from build123d import *

# Parameters (mm, degrees)
SKETCH1_W                 = 97.7
SKETCH1_H                 = 140
BOSS_EXTRUDE1_DEPTH       = 6.35
FILLET1_R                 = 10
CUT_EXTRUDE1_DEPTH        = 6.35
SKETCH5_R                 = 2.4
CUT_EXTRUDE2_DEPTH        = 6.35
F_5_0MM_DOWEL_HOLE1_D     = 5
F_5_0MM_DOWEL_HOLE1_DEPTH = 10
F_5_0MM_DOWEL_HOLE1_TIP   = 1.502151548


with BuildPart() as part:
    # Sketch1 → Boss-Extrude1 (new body)
    with BuildSketch(Plane(origin=(0, 0, 0), x_dir=(1, 0, 0), z_dir=(0, 1, 0))):
        with Locations((3.993769968, 7.891373802)):
            Rectangle(SKETCH1_W, SKETCH1_H)
    extrude(amount=BOSS_EXTRUDE1_DEPTH)

    # Fillet1
    fillet1_edges = [part.edges().sort_by_distance(p)[0] for p in [
        (-44.856230032, 3.175, -77.891373802),
        (-44.856230032, 3.175, 62.108626198),
    ]]
    fillet(fillet1_edges, radius=FILLET1_R)

    # Sketch3 → Cut-Extrude1 (cut)
    with BuildSketch(Plane(origin=(0, 6.35, 0), x_dir=(1, 0, 0), z_dir=(0, 1, 0))):
        Polygon((-29.556230032, 63.491373802), (-29.556230032, -40), (34.243769968, -40), (34.343769968, 63.391373802), align=None)
    extrude(amount=-CUT_EXTRUDE1_DEPTH, mode=Mode.SUBTRACT)

    # Sketch5 → Cut-Extrude2 (cut)
    with BuildSketch(Plane(origin=(0, 6.35, 0), x_dir=(1, 0, 0), z_dir=(0, 1, 0))):
        with Locations((-36.656230032, 40.391373802)):
            Circle(SKETCH5_R)
        with Locations((-36.656230032, 24.391373802)):
            Circle(SKETCH5_R)
        with Locations((-36.656230032, -8.608626198)):
            Circle(SKETCH5_R)
        with Locations((-36.656230032, -24.608626198)):
            Circle(SKETCH5_R)
        with Locations((-36.656230032, -16.608626198)):
            Circle(SKETCH5_R)
        with Locations((-36.656230032, 32.391373802)):
            Circle(SKETCH5_R)
    extrude(amount=-CUT_EXTRUDE2_DEPTH, mode=Mode.SUBTRACT)

    # Ø5.0mm Dowel Hole1
    with Locations(Plane(origin=(0, 6.35, 0), x_dir=(1, 0, 0), z_dir=(0, 1, 0))):
        with Locations((46.493769968, 45.888131535), (46.493769968, 15.888131535), (46.493769968, -14.111868465), (46.493769968, -44.111868465)):
            Hole(F_5_0MM_DOWEL_HOLE1_D / 2, depth=F_5_0MM_DOWEL_HOLE1_DEPTH)
            with Locations((0, 0, -(F_5_0MM_DOWEL_HOLE1_DEPTH + F_5_0MM_DOWEL_HOLE1_TIP / 2))):  # 118° drill point
                Cone(0, F_5_0MM_DOWEL_HOLE1_D / 2, F_5_0MM_DOWEL_HOLE1_TIP, mode=Mode.SUBTRACT)


solid = part.part
Could you check a few things on this model? Use its own coordinates, in mm. Give positions to 0.01 mm unless a question says otherwise; leave off trailing zeros. Order: outer loops, then holes, each group sorted by start corner. A loop starts at its lowest first (then second) coordinate and runs counter-clockwise, first axis right, second up.
1. We'd pull the mould along X, two halves only. Please class faces 1 (the cylindrical face through (44.184, 3.131, -14.931)), 2 (the flat face through (36, 6.35, -9)), 3 (the flat face through (-44.856, 3, -7)): pulls with the +X half, pulls with the -X half, needs draft (parallel to the pull), parting line crosses it, or undercut.
2. Suppose I cut it at B-B (y = 3). Give the number of separate pieces and of enclosed holes in the cut face, plus the area to 3 significant figures.
3. Suppose I cut it at A-A (x = -18). List the corners of the cut face in (y, z) for me, plus the area to 3 significant figures.
4. Will these pins go through, and if not, where does the flat tip stop? P1, Ø4, axis at x = 46.49, z = -15.89, coming from the +Y side; P2, Ø6, axis at x = -36.66, z = -32.39, coming from the -Y side.
5. I need wall thicknesses on L1, parallel to Z at x = 46.5, y = 3.75; L2, parallel to Z at x = -13, y = 0.5; L3, parallel to X at y = 6, z = -55. Which ranges of each line are inside material? Lowest first, please.
6. Suppose I cut it at C-C (x = 12.5). List the corners of the cut face in (y, z) for me, plus the area to 3 significant figures.
Solved:
1. face 1: undercut
1. face 2: needs draft
1. face 3: pulls with the -X half
2. separate pieces: 1
2. enclosed holes: 11
2. area: 6,840 mm2
3. outline: (0, -77.89) - (6.35, -77.89) - (6.35, -63.47) - (0, -63.47) - close; (0, 40) - (6.35, 40) - (6.35, 62.11) - (0, 62.11) - close
3. area: 232 mm2
4. P1: passes through
4. P2: stops at y = 0
5. L1: z = -77.89 to -48.39, -43.39 to -18.39, -13.39 to 11.61, 16.61 to 41.61, 46.61 to 62.11
5. L2: z = -77.89 to -63.47, 40 to 62.11
5. L3: x = -44.86 to -29.56, 34.34 to 52.84
6. outline: (0, -77.89) - (6.35, -77.89) - (6.35, -63.43) - (0, -63.43) - close; (0, 40) - (6.35, 40) - (6.35, 62.11) - (0, 62.11) - close
6. area: 232 mm2
